Can you work these out from the drawing? Everything is in mm from the part's minimum corner. Round coordinates to 2 decimals unless told otherwise and drop trailing zeros. Loops run counter-clockwise (first coordinate to the right, second up) from the corner with the lowest first, then second, coordinate; pieces in that order, holes last. Notation, with made-up numbers: M 2.5,-35.5 L 52.5,-35.5 A35 ccw 52.5,1.5 Z; hole C -14,-19 d9. An arc over 180 degrees is marked long. Use a Markdown table: item, result.
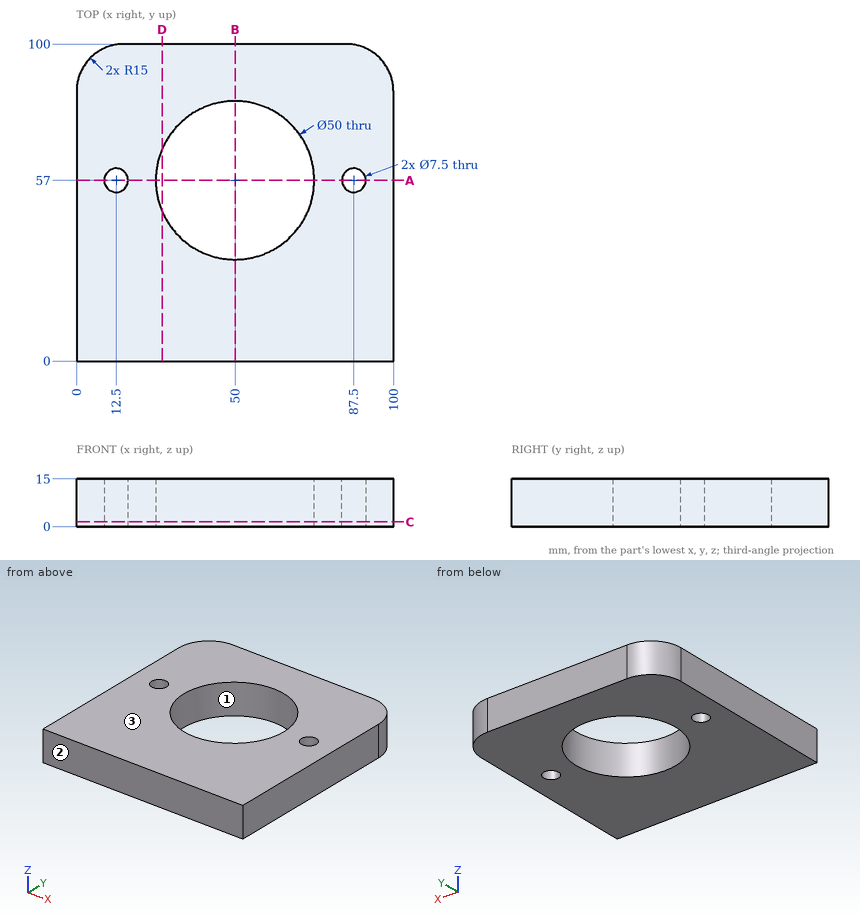
1. Imagine slicing it at D-D, the plane x = 27. Write out the boundary of the cut face in (y, z), then the cut area to 3 significant figures.
Answer sheet:
| item | result |
|---|---|
| outline | M 0,0 L 47.2,0 L 47.2,15 L 0,15 Z; M 66.8,0 L 100,0 L 100,15 L 66.8,15 Z |
| area | 1,210 mm2 |
2. Imagine slicing it at B-B, the plane x = 50. Write out the boundary of the cut face in (y, z).
Answer sheet:
| item | result |
|---|---|
| outline | M 0,0 L 32,0 L 32,15 L 0,15 Z; M 82,0 L 100,0 L 100,15 L 82,15 Z |
3. I need wall thicknesses on probe 1 along Y at (x, z) = (50, 10); probe 2 along X at (y, z) = (55.5, 13.5); probe 3 along Y at (x, z) = (12.5, 3.75). Which ranges of each line are inside material? Lowest first, please. Write a range as from..to.
Answer sheet:
| item | result |
|---|---|
| probe 1 | 0..32, 82..100 |
| probe 2 | 0..9.06, 15.94..25.05, 74.95..84.06, 90.94..100 |
| probe 3 | 0..53.25, 60.75..99.79 |
4. Imagine slicing it at C-C, the plane z = 1.5. Write out the boundary of the cut face in (x, y), then the cut area to 3 significant figures.
Answer sheet:
| item | result |
|---|---|
| outline | M 0,0 L 100,0 L 100,85 A15 ccw 85,100 L 15,100 A15 ccw 0,85 Z; hole C 12.5,57 d7.5; hole C 50,57 d50; hole C 87.5,57 d7.5 |
| area | 7,850 mm2 |
5. Imagine slicing it at A-A, the plane y = 57. Write out the boundary of the cut face in (x, z).
Answer sheet:
| item | result |
|---|---|
| outline | M 0,0 L 8.75,0 L 8.75,15 L 0,15 Z; M 16.25,0 L 25,0 L 25,15 L 16.25,15 Z; M 75,0 L 83.75,0 L 83.75,15 L 75,15 Z; M 91.25,0 L 100,0 L 100,15 L 91.25,15 Z |
6. For pin 1 Ø10 at (x, y) = (12.5, 57) entering from -Z, with a flat end and sliding along its axis, tell me the tip position at first contact or that it passes through.
Answer sheet:
| item | result |
|---|---|
| pin 1 | z = 0 |
7. We'd pull the mould along Y, two halves only. Please class the marked faces 1, 2 and 3: +Y half, -Y half, draft (parallel to the pull), parting line (faces both ways), or undercut.
Answer sheet:
| item | result |
|---|---|
| face 1 | undercut |
| face 2 | -Y half |
| face 3 | draft |
